Verification items for the finished model (mm, model axes). A direction names the side the tool comes from. Round coordinates to 2 decimals unless told otherwise and drop trailing zeros. Write each loop counter-clockwise with the first axis right and the second up, starting at its lowest first coordinate (ties: lowest second). Pieces come first, ordered by that corner, then holes. Notation, with made-up numbers: M 51.5,44 L 81.5,44 A15 ccw 81.5,64 Z; hole C -10.75,-6.75 d4. An arc over 180 degrees is marked long. One line per item, written item: value. Start each with the question number.
Item 1: Tool access check on faces 5 (the face through (-19.279, -24, 36)), 6 (the face through (23.3, 26.4, 73.66)), 7 (the face through (17.01, -27.26, 36.31)). Record the directions out of +Z, -Z, +X, -X, +Y, -Y that give a thin tool (end or side, any length) a straight path to the whole face; none if there is none.
Item 2: Thickness scan on probe 1 along Z at (x, y) = (10.5, -13); probe 2 along Y at (x, z) = (-8, 23.5) (3 decimals); probe 3 along Z at (x, y) = (22.5, 6.5). Record the ranges inside material, lowest first. Write a range as from..to.
Item 3: Gauge pin test, flat ends, axial feed: pin 1 (1.5 mm diameter, centred on x = 21.5, y = 25.5, fed in from -Z); pin 2 (1.7 mm diameter, centred on x = 0.5, z = 91, fed in from +Y); pin 3 (1.9 mm diameter, centred on y = -23.5, z = 30, fed in from +X). Record the tip position at first contact, or that the pin passes through.
Item 4: Section check D-D, the plane y = 60.5. Record the cut outline in (x, z) (3 decimals), then the cut area to 3 significant figures.
Item 5: Draft check along Y on faces 1 (the face through (-26, -25, 73.66)), 2 (the face through (25.97, -24.59, 76.24)), 3 (the face through (0, -28.575, 40)), 4 (the face through (0, 28.575, 40)). Enter one of: +Y half, -Y half, draft (parallel to the pull), parting line (faces both ways), or undercut.
Item 6: Section check B-B, the plane y = 0. Record the cut outline in (x, z) (3 decimals).
Item 7: Section check A-A, the plane z = 28.5. Record the cut outline in (x, y) (3 decimals).
Item 8: Section check C-C, the plane x = -6.5. Record the cut outline in (y, z) (3 decimals).
from build123d import *

# Parameters (mm, degrees)
SKETCH1_W           = 57.15
SKETCH1_H           = 78.74
BOSS_EXTRUDE1_DEPTH = 57.15
CUT_EXTRUDE1_DEPTH  = 73.66
CUT_EXTRUDE2_DEPTH  = 73.66
CUT_EXTRUDE3_DEPTH  = 73.66
CUT_EXTRUDE4_DEPTH  = 73.66
CUT_EXTRUDE5_DEPTH  = 73.66
CUT_EXTRUDE6_DEPTH  = 73.66
CUT_EXTRUDE7_DEPTH  = 73.66
CUT_EXTRUDE8_DEPTH  = 73.66
SKETCH10_R          = 19.05
BOSS_EXTRUDE2_DEPTH = 1.524
SKETCH11_R          = 3.175
BOSS_EXTRUDE3_DEPTH = 19.05
CUT_EXTRUDE9_DEPTH  = 14.986
SKETCH13_W          = 0.635
SKETCH13_H          = 85.725
SKETCH14_W          = 0.635
SKETCH14_H          = 85.725
SKETCH15_W          = 0.635
SKETCH15_H          = 85.725
SKETCH16_W          = 0.635
SKETCH16_H          = 85.725
HOLE1_D             = 5.08
HOLE1_DEPTH         = 25.654
HOLE2_D             = 5.08
HOLE2_DEPTH         = 25.654
HOLE3_D             = 5.08
HOLE3_DEPTH         = 25.654
HOLE4_D             = 5.08
HOLE4_DEPTH         = 25.654
CHAMFER1_SIZE       = 0.254
FILLET1_R           = 2.54
FILLET2_R           = 2.54
FILLET3_R           = 2.54
FILLET4_R           = 2.54
FILLET5_R           = 2.54
FILLET6_R           = 2.54
FILLET7_R           = 2.54
FILLET8_R           = 2.54


with BuildPart() as part:
    # Sketch1 → Boss-Extrude1 (new body)
    with BuildSketch(Plane.XZ.offset(28.575)):
        with Locations((0, 39.37)):
            Rectangle(SKETCH1_W, SKETCH1_H)
    extrude(amount=-BOSS_EXTRUDE1_DEPTH)

    # Sketch2 → Cut-Extrude1 (cut)
    with BuildSketch(Plane(origin=(0, 0, 0), x_dir=(-1, 0, 0), z_dir=(0, 0, -1))):
        with BuildLine():
            Line((-28.575, -28.575), (-14.692533342, -28.575))
            ThreePointArc((-14.692533342, -28.575), (-22.720047986, -22.720047986), (-28.575, -14.692533342))
            Line((-28.575, -14.692533342), (-28.575, -28.575))
        make_face()
    extrude(amount=-CUT_EXTRUDE1_DEPTH, mode=Mode.SUBTRACT)

    # Sketch3 → Cut-Extrude2 (cut)
    with BuildSketch(Plane(origin=(0, 0, 0), x_dir=(-1, 0, 0), z_dir=(0, 0, -1))):
        with BuildLine():
            Line((-19.2786, -25.7048), (-19.2786, -19.2786))
            Line((-19.2786, -19.2786), (-25.7048, -19.2786))
            ThreePointArc((-25.7048, -19.2786), (-22.720047986, -22.720047986), (-19.2786, -25.7048))
        make_face()
    extrude(amount=-CUT_EXTRUDE2_DEPTH, mode=Mode.SUBTRACT)

    # Sketch4 → Cut-Extrude3 (cut)
    with BuildSketch(Plane(origin=(0, 0, 0), x_dir=(-1, 0, 0), z_dir=(0, 0, -1))):
        with BuildLine():
            Line((-28.575, 28.575), (-28.575, 14.692533342))
            ThreePointArc((-28.575, 14.692533342), (-22.720047986, 22.720047986), (-14.692533342, 28.575))
            Line((-14.692533342, 28.575), (-28.575, 28.575))
        make_face()
    extrude(amount=-CUT_EXTRUDE3_DEPTH, mode=Mode.SUBTRACT)

    # Sketch5 → Cut-Extrude4 (cut)
    with BuildSketch(Plane(origin=(0, 0, 0), x_dir=(-1, 0, 0), z_dir=(0, 0, -1))):
        with BuildLine():
            Line((-25.7048, 19.2786), (-19.2786, 19.2786))
            Line((-19.2786, 19.2786), (-19.2786, 25.7048))
            ThreePointArc((-19.2786, 25.7048), (-22.720047986, 22.720047986), (-25.7048, 19.2786))
        make_face()
    extrude(amount=-CUT_EXTRUDE4_DEPTH, mode=Mode.SUBTRACT)

    # Sketch6 → Cut-Extrude5 (cut)
    with BuildSketch(Plane(origin=(0, 0, 0), x_dir=(-1, 0, 0), z_dir=(0, 0, -1))):
        with BuildLine():
            Line((28.575, 28.575), (14.692533342, 28.575))
            ThreePointArc((14.692533342, 28.575), (22.720047986, 22.720047986), (28.575, 14.692533342))
            Line((28.575, 14.692533342), (28.575, 28.575))
        make_face()
    extrude(amount=-CUT_EXTRUDE5_DEPTH, mode=Mode.SUBTRACT)

    # Sketch7 → Cut-Extrude6 (cut)
    with BuildSketch(Plane(origin=(0, 0, 0), x_dir=(-1, 0, 0), z_dir=(0, 0, -1))):
        with BuildLine():
            Line((19.2786, 25.7048), (19.2786, 19.2786))
            Line((19.2786, 19.2786), (25.7048, 19.2786))
            ThreePointArc((25.7048, 19.2786), (22.720047986, 22.720047986), (19.2786, 25.7048))
        make_face()
    extrude(amount=-CUT_EXTRUDE6_DEPTH, mode=Mode.SUBTRACT)

    # Sketch8 → Cut-Extrude7 (cut)
    with BuildSketch(Plane(origin=(0, 0, 0), x_dir=(-1, 0, 0), z_dir=(0, 0, -1))):
        with BuildLine():
            Line((28.575, -28.575), (28.575, -14.692533342))
            ThreePointArc((28.575, -14.692533342), (22.720047986, -22.720047986), (14.692533342, -28.575))
            Line((14.692533342, -28.575), (28.575, -28.575))
        make_face()
    extrude(amount=-CUT_EXTRUDE7_DEPTH, mode=Mode.SUBTRACT)

    # Sketch9 → Cut-Extrude8 (cut)
    with BuildSketch(Plane(origin=(0, 0, 0), x_dir=(-1, 0, 0), z_dir=(0, 0, -1))):
        with BuildLine():
            Line((25.7048, -19.2786), (19.2786, -19.2786))
            Line((19.2786, -19.2786), (19.2786, -25.7048))
            ThreePointArc((19.2786, -25.7048), (22.720047986, -22.720047986), (25.7048, -19.2786))
        make_face()
    extrude(amount=-CUT_EXTRUDE8_DEPTH, mode=Mode.SUBTRACT)

    # Sketch10 → Boss-Extrude2 (add)
    with BuildSketch(Plane.XY.offset(78.74)):
        Circle(SKETCH10_R)
    extrude(amount=BOSS_EXTRUDE2_DEPTH)

    # Sketch11 → Boss-Extrude3 (add)
    with BuildSketch(Plane.XY.offset(80.264)):
        Circle(SKETCH11_R)
    extrude(amount=BOSS_EXTRUDE3_DEPTH)

    # Sketch12 → Cut-Extrude9 (cut)
    with BuildSketch(Plane.XY.offset(99.314)):
        with BuildLine():
            Line((-1.722711816, 2.667), (1.722711816, 2.667))
            ThreePointArc((1.722711816, 2.667), (0, 3.175), (-1.722711816, 2.667))
        make_face()
    extrude(amount=-CUT_EXTRUDE9_DEPTH, mode=Mode.SUBTRACT)

    # Sketch13 → Revolve1 (revolve)
    with BuildSketch(Plane(origin=(0, 0, 12.7), x_dir=(-1, 0, 0), z_dir=(0, 0, -1))):
        with Locations((1.7145, 71.4375)):
            Rectangle(SKETCH13_W, SKETCH13_H)
    revolve(axis=Axis((-2.032, 28.575, 12.7), (0, 1, 0)))

    # Sketch14 → Revolve2 (revolve)
    with BuildSketch(Plane(origin=(0, 0, 12.7), x_dir=(-1, 0, 0), z_dir=(0, 0, -1))):
        with Locations((-2.3495, 71.4375)):
            Rectangle(SKETCH14_W, SKETCH14_H)
    revolve(axis=Axis((2.032, 28.575, 12.7), (0, 1, 0)))

    # Sketch15 → Revolve3 (revolve)
    with BuildSketch(Plane(origin=(0, 0, 14.732), x_dir=(-1, 0, 0), z_dir=(0, 0, -1))):
        with Locations((-0.3175, 71.4375)):
            Rectangle(SKETCH15_W, SKETCH15_H)
    revolve(axis=Axis((0, 28.575, 14.732), (0, 1, 0)))

    # Sketch16 → Revolve4 (revolve)
    with BuildSketch(Plane(origin=(0, 0, 10.668), x_dir=(-1, 0, 0), z_dir=(0, 0, -1))):
        with Locations((-0.3175, 71.4375)):
            Rectangle(SKETCH16_W, SKETCH16_H)
    revolve(axis=Axis((0, 28.575, 10.668), (0, 1, 0)))

    # Hole1
    with Locations(Plane(origin=(0, 0, 73.66), x_dir=(-1, 0, 0), z_dir=(0, 0, -1))):
        with Locations((23.622, -23.622)):
            Hole(HOLE1_D / 2, depth=HOLE1_DEPTH)

    # Hole2
    with Locations(Plane(origin=(0, 0, 73.66), x_dir=(-1, 0, 0), z_dir=(0, 0, -1))):
        with Locations((23.622, 23.622)):
            Hole(HOLE2_D / 2, depth=HOLE2_DEPTH)

    # Hole3
    with Locations(Plane(origin=(0, 0, 73.66), x_dir=(-1, 0, 0), z_dir=(0, 0, -1))):
        with Locations((-23.622, 23.622)):
            Hole(HOLE3_D / 2, depth=HOLE3_DEPTH)

    # Hole4
    with Locations(Plane(origin=(0, 0, 73.66), x_dir=(-1, 0, 0), z_dir=(0, 0, -1))):
        with Locations((-23.622, -23.622)):
            Hole(HOLE4_D / 2, depth=HOLE4_DEPTH)

    # Chamfer1
    chamfer1_edges = [part.edges().sort_by_distance(p)[0] for p in [
        (-1.51838977, -2.78838977, 99.314),
    ]]
    chamfer(chamfer1_edges, length=CHAMFER1_SIZE)

    # Fillet1
    fillet1_edges = [part.edges().sort_by_distance(p)[0] for p in [
        (-28.575, 28.575, 76.2),
    ]]
    fillet(fillet1_edges, radius=FILLET1_R)

    # Fillet2
    fillet2_edges = [part.edges().sort_by_distance(p)[0] for p in [
        (-28.575, -28.575, 76.2),
    ]]
    fillet(fillet2_edges, radius=FILLET2_R)

    # Fillet3
    fillet3_edges = [part.edges().sort_by_distance(p)[0] for p in [
        (28.575, 28.575, 76.2),
    ]]
    fillet(fillet3_edges, radius=FILLET3_R)

    # Fillet4
    fillet4_edges = [part.edges().sort_by_distance(p)[0] for p in [
        (-19.2786, 19.2786, 36.83),
    ]]
    fillet(fillet4_edges, radius=FILLET4_R)

    # Fillet5
    fillet5_edges = [part.edges().sort_by_distance(p)[0] for p in [
        (28.575, -28.575, 76.2),
    ]]
    fillet(fillet5_edges, radius=FILLET5_R)

    # Fillet6
    fillet6_edges = [part.edges().sort_by_distance(p)[0] for p in [
        (19.2786, -19.2786, 36.83),
    ]]
    fillet(fillet6_edges, radius=FILLET6_R)

    # Fillet7
    fillet7_edges = [part.edges().sort_by_distance(p)[0] for p in [
        (19.2786, 19.2786, 36.83),
    ]]
    fillet(fillet7_edges, radius=FILLET7_R)

    # Fillet8
    fillet8_edges = [part.edges().sort_by_distance(p)[0] for p in [
        (-19.2786, -19.2786, 36.83),
    ]]
    fillet(fillet8_edges, radius=FILLET8_R)


solid = part.part
Response values:
1. face 5: -Z, -X, -Y
1. face 6: -Z, +X, +Y
1. face 7: -Z, +X, -Y
2. probe 1: z = 0..80.26
2. probe 2: y = -28.575..28.575
2. probe 3: z = 0..78.74
3. pin 1: stops at z = 73.66
3. pin 2: stops at y = 2.67
3. pin 3: stops at x = 19.28
4. outline: C -2.032,12.7 d1.27; C 0,10.668 d1.27; C 0,14.732 d1.27; C 2.032,12.7 d1.27
4. area: 5.07 mm2
5. face 1: draft
5. face 2: undercut
5. face 3: -Y half
5. face 4: +Y half
6. outline: M -28.575,0 L 28.575,0 L 28.575,78.74 L 19.05,78.74 L 19.05,80.264 L 3.175,80.264 L 3.175,99.06 L 2.921,99.314 L -2.921,99.314 L -3.175,99.06 L -3.175,80.264 L -19.05,80.264 L -19.05,78.74 L -28.575,78.74 Z
7. outline: M -28.575,-14.693 A32.131 ccw -25.705,-19.279 L -21.819,-19.279 A2.54 cw -19.279,-21.819 L -19.279,-25.705 A32.131 ccw -14.693,-28.575 L 14.693,-28.575 A32.131 ccw 19.279,-25.705 L 19.279,-21.819 A2.54 cw 21.819,-19.279 L 25.705,-19.279 A32.131 ccw 28.575,-14.693 L 28.575,14.693 A32.131 ccw 25.705,19.279 L 21.819,19.279 A2.54 cw 19.279,21.819 L 19.279,25.705 A32.131 ccw 14.693,28.575 L -14.693,28.575 A32.131 ccw -19.279,25.705 L -19.279,21.819 A2.54 cw -21.819,19.279 L -25.705,19.279 A32.131 ccw -28.575,14.693 Z
8. outline: M -28.575,0 L 28.575,0 L 28.575,78.74 L 17.907,78.74 L 17.907,80.264 L -17.907,80.264 L -17.907,78.74 L -28.575,78.74 Z
